Part model, mm, in its own coordinate system. A direction names the side the tool comes from. Round coordinates to 2 decimals unless told otherwise and drop trailing zeros. Loops run counter-clockwise (first coordinate to the right, second up) from the corner with the lowest first, then second, coordinate; pieces in that order, holes last. Notation, with made-up numbers: (53, 36.5) -> (73, 36.5) arc R13 ccw to (73, 56.5) -> close; hole circle Ø8 at (83.5, -39.5). An arc over 180 degrees is marked (long way). Use a Markdown table: item, result. Add a question column.
Item 1: Cut at D-D, the plane y = 135. List the corners of the cut face in (x, z).
Item 2: Cut at A-A, the plane y = 0. List the corners of the cut face in (x, z).
Item 3: Cut at B-B, the plane y = -171. List the corners of the cut face in (x, z).
Item 4: Which spindle directions (+Z, -Z, +X, -X, +Y, -Y) get a long thin tool onto all of the face, cutting with end or side? Do faces 1 (the face through (-3, 3, 0)), 2 (the face through (-90.17, 63, 1.52)). Say none if no direction does.
Item 5: Flat gauge pins, fed straight in: pin 1 (1.5 mm diameter, centred on x = 58.5, z = 2, fed in from -Y); pin 2 (1.5 mm diameter, centred on x = -68.5, z = 1, fed in from -Y). Where does each tip first touch, or does it go through?
Item 6: Two-plate mould, pull along Y, no slides. Class faces 3 (the face through (190.764, 60.075, 1.479)), 4 (the face through (-106.426, 74.657, 1.521)), 5 (the face through (-3, 3, 3)): pulls with the +Y half, pulls with the -Y half, needs draft (parallel to the pull), parting line crosses it, or undercut.
Item 7: Cut at C-C, the plane z = 1.8. State how many separate pieces and enclosed holes the cut face has, plus the area to 3 significant figures.
Item 8: Probe line 1 (X direction, y = 84, z = 0.4); line 2 (X direction, y = 70, z = 1.65); line 3 (X direction, y = 9, z = 0.35). List the from-to ranges inside material, lowest first. Write a range as [from, to].
```python
from build123d import *

# Parameters (mm, degrees)
SKETCH1_R           = 200
BOSS_EXTRUDE2_DEPTH = 3
SKETCH9_R           = 3.5
CUT_EXTRUDE8_DEPTH  = 3
CIRPATTERN5_COUNT   = 3
SKETCH15_R          = 2
CUT_EXTRUDE13_DEPTH = 3
SKETCH17_R          = 3.5
CUT_EXTRUDE15_DEPTH = 3
CIRPATTERN7_COUNT   = 3
CUT_EXTRUDE16_DEPTH = 3
CUT_EXTRUDE17_DEPTH = 3
SKETCH20_R          = 1.6
CUT_EXTRUDE18_DEPTH = 3
FILLET1_R           = 2
SKETCH21_R          = 2
CUT_EXTRUDE19_DEPTH = 3


with BuildPart() as part:
    # Sketch1 → Boss-Extrude2 (new body)
    with BuildSketch(Plane.XY):
        Circle(SKETCH1_R)
    extrude(amount=BOSS_EXTRUDE2_DEPTH)

    # Sketch9 → Cut-Extrude8 (cut)
    with BuildSketch(Plane.XY.offset(3)):
        with Locations((-56.715390309, 146.233937587)):
            Circle(SKETCH9_R)
        with Locations((-98.284609691, 122.233937587)):
            Circle(SKETCH9_R)
    cut_extrude8 = extrude(amount=-CUT_EXTRUDE8_DEPTH, mode=Mode.SUBTRACT)

    # CirPattern5: Cut-Extrude8 ×3 about axis
    cirpattern5_axis = Axis((0, 0, 0), (0, 0, 1))
    for i in range(1, CIRPATTERN5_COUNT):
        add(cut_extrude8.rotate(cirpattern5_axis, i * 360 / CIRPATTERN5_COUNT), mode=Mode.SUBTRACT)

    # Sketch15 → Cut-Extrude13 (cut)
    with BuildSketch(Plane.XY.offset(3)):
        with Locations((20, 85)):
            Circle(SKETCH15_R)
        with Locations((60, 85)):
            Circle(SKETCH15_R)
    extrude(amount=-CUT_EXTRUDE13_DEPTH, mode=Mode.SUBTRACT)

    # Sketch17 → Cut-Extrude15 (cut)
    with BuildSketch(Plane.XY.offset(3)):
        with Locations((-84.532410842, 88.488821425)):
            Circle(SKETCH17_R)
        with Locations((-112.064079787, 49.169523299)):
            Circle(SKETCH17_R)
        with Locations((-56.715390309, 146.233937587)):
            Circle(SKETCH17_R)
        with Locations((-98.284609691, 122.233937587)):
            Circle(SKETCH17_R)
        Polygon((-112.225530121, 66.373416283), (-95.842489235, 54.901887556), (-84.370960508, 71.284928442), (-100.754001394, 82.756457169), align=None)
        with BuildLine():
            Line((-79.907686902, 60.22467579), (-73.354470547, 55.636064299))
            ThreePointArc((-73.354470547, 55.636064299), (-72.49495592, 50.761514617), (-77.369505602, 49.901999989))
            Line((-77.369505602, 49.901999989), (-83.922721956, 54.49061148))
            ThreePointArc((-83.922721956, 54.49061148), (-84.782236584, 59.365161162), (-79.907686902, 60.22467579))
        make_face()
        with BuildLine():
            Line((-112.673768673, 83.167733244), (-119.226985028, 87.756344735))
            ThreePointArc((-119.226985028, 87.756344735), (-124.10153471, 86.896830107), (-123.242020082, 82.022280425))
            Line((-123.242020082, 82.022280425), (-116.688803728, 77.433668934))
            ThreePointArc((-116.688803728, 77.433668934), (-111.814254045, 78.293183562), (-112.673768673, 83.167733244))
        make_face()
    cut_extrude15 = extrude(amount=-CUT_EXTRUDE15_DEPTH, mode=Mode.SUBTRACT)

    # CirPattern7: Cut-Extrude15 ×3 about axis
    cirpattern7_axis = Axis((0, 0, 0), (0, 0, 1))
    for i in range(1, CIRPATTERN7_COUNT):
        add(cut_extrude15.rotate(cirpattern7_axis, i * 360 / CIRPATTERN7_COUNT), mode=Mode.SUBTRACT)

    # Sketch18 → Cut-Extrude16 (cut)
    with BuildSketch(Plane.XY.offset(3)):
        with BuildLine():
            Line((-5, 30), (-5, -50))
            ThreePointArc((-5, -50), (-10, -55), (-15, -50))
            Line((-15, -50), (-15, 30))
            ThreePointArc((-15, 30), (-10, 35), (-5, 30))
        make_face()
    extrude(amount=-CUT_EXTRUDE16_DEPTH, mode=Mode.SUBTRACT)

    # Sketch19 → Cut-Extrude17 (cut)
    with BuildSketch(Plane.XY.offset(3)):
        with BuildLine():
            Line((30, -90), (110, -90))
            ThreePointArc((110, -90), (115, -95), (110, -100))
            Line((110, -100), (30, -100))
            ThreePointArc((30, -100), (25, -95), (30, -90))
        make_face()
    extrude(amount=-CUT_EXTRUDE17_DEPTH, mode=Mode.SUBTRACT)

    # Sketch20 → Cut-Extrude18 (cut)
    with BuildSketch(Plane.XY.offset(3)):
        with Locations((-57.987394178, 121.9)):
            Circle(SKETCH20_R)
        with Locations((-10, 120.8)):
            Circle(SKETCH20_R)
        with Locations((-53.287394178, 70)):
            Circle(SKETCH20_R)
        with Locations((-25.387394178, 70)):
            Circle(SKETCH20_R)
    extrude(amount=-CUT_EXTRUDE18_DEPTH, mode=Mode.SUBTRACT)

    # Fillet1
    fillet1_edges = [part.edges().sort_by_distance(p)[0] for p in [
        (-1.368299576, -130.376868179, 1.5),
        (-21.292193538, -128.633753324, 1.5),
        (-19.549078683, -108.709859363, 1.5),
        (0.374815279, -110.452974218, 1.5),
        (113.593829697, 64.003451897, 1.5),
        (122.046194932, 45.877296156, 1.5),
        (103.920039191, 37.424930921, 1.5),
        (95.467673957, 55.551086662, 1.5),
        (-112.225530121, 66.373416283, 1.5),
        (-100.754001394, 82.756457169, 1.5),
        (-84.370960508, 71.284928442, 1.5),
        (-95.842489235, 54.901887556, 1.5),
    ]]
    fillet(fillet1_edges, radius=FILLET1_R)

    # Sketch21 → Cut-Extrude19 (cut)
    with BuildSketch(Plane.XY.offset(3)):
        with Locations((-154, 10)):
            Circle(SKETCH21_R)
        with Locations((-40, 10)):
            Circle(SKETCH21_R)
        with Locations((-154, -74)):
            Circle(SKETCH21_R)
        with Locations((-40, -74)):
            Circle(SKETCH21_R)
    extrude(amount=-CUT_EXTRUDE19_DEPTH, mode=Mode.SUBTRACT)


solid = part.part
```
A:
| question | item | result |
|---|---|---|
| 1 | outline | (-147.56, 0) -> (147.56, 0) -> (147.56, 3) -> (-147.56, 3) -> close |
| 2 | outline | (-200, 0) -> (-15, 0) -> (-15, 3) -> (-200, 3) -> close; (-5, 0) -> (200, 0) -> (200, 3) -> (-5, 3) -> close |
| 3 | outline | (-103.73, 0) -> (103.73, 0) -> (103.73, 3) -> (-103.73, 3) -> close |
| 4 | face 1 | -Z, +X, -X, +Y, -Y |
| 4 | face 2 | +Z, -Z |
| 5 | pin 1 | stops at y = -191.48 |
| 5 | pin 2 | stops at y = -188.18 |
| 6 | face 3 | parting line crosses it |
| 6 | face 4 | undercut |
| 6 | face 5 | needs draft |
| 7 | separate pieces | 1 |
| 7 | enclosed holes | 33 |
| 7 | area | 122,000 mm^2 |
| 8 | line 1 | x = [-181.5, -124.62], [-113.86, 18.27], [21.73, 58.27], [61.73, 181.5] |
| 8 | line 2 | x = [-187.35, -109.69], [-85.32, -54.89], [-51.69, -26.99], [-23.79, 96.13], [101.1, 187.35] |
| 8 | line 3 | x = [-199.8, -155.73], [-152.27, -41.73], [-38.27, -15], [-5, 199.8] |
